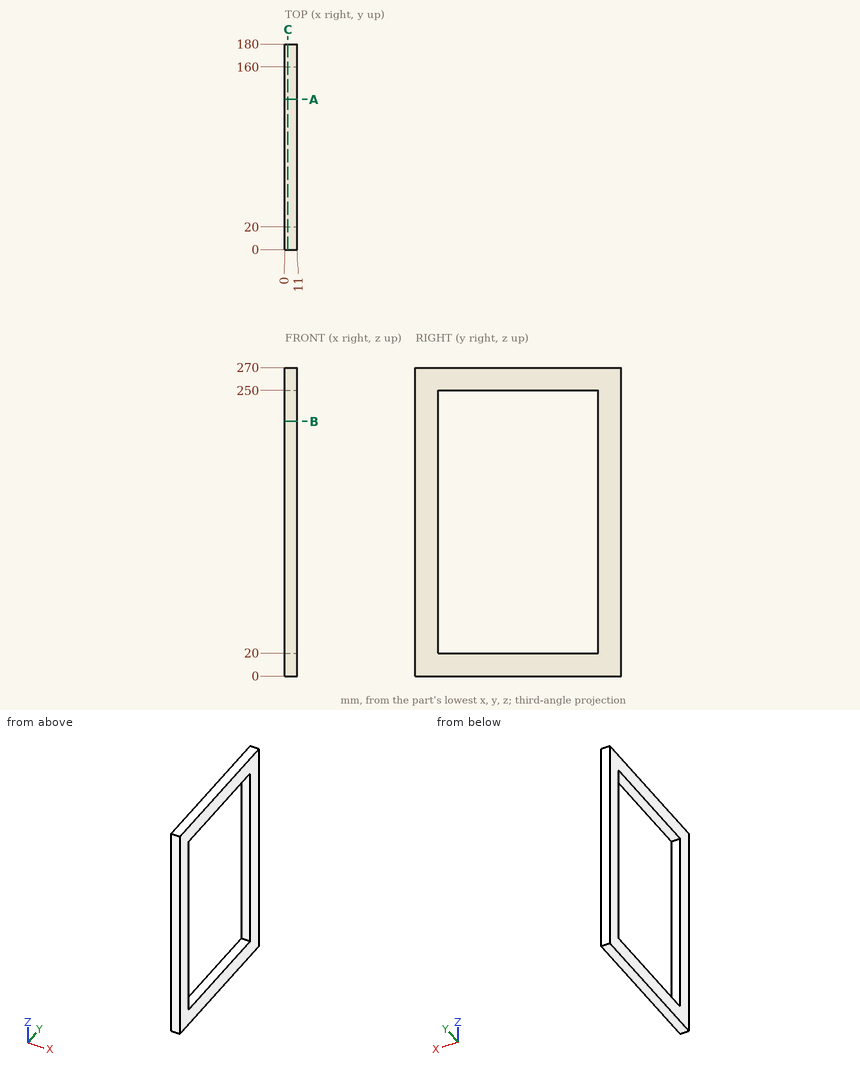
Part print with two shaded views. Sizes in mm from the minimum x, y, z corner. Round coordinates to 2 decimals unless told otherwise and drop trailing zeros. Order: outer loops, then holes, each group sorted by start corner. A loop starts at its lowest first (then second) coordinate and runs counter-clockwise, first axis right, second up. Notation, with made-up numbers: (27, 23) - (58, 23) arc R31 ccw to (58, 53) - close; hole circle Ø8 at (31.25, 62.25). An arc over 180 degrees is marked (long way). Answer in a Markdown table with one row per item. Add a question column.
(1) Probe L1, parallel to Z at x = 9.5, y = 116; L2, parallel to Y at x = 10, z = 138. List the from-to ranges inside material, lowest first. Write a range as [from, to].
(2) Band-saw the part on A-A on y = 131.5. List the corners of the cut face in (x, z), and give its area (3 significant figures).
(3) Band-saw the part on C-C on x = 2.5. List the corners of the cut face in (y, z), and give its area (3 significant figures).
(4) Band-saw the part on B-B on z = 223. List the corners of the cut face in (x, y).
Data:
| question | item | result |
|---|---|---|
| 1 | L1 | z = [0, 20], [250, 270] |
| 1 | L2 | y = [0, 20], [160, 180] |
| 2 | outline | (0, 0) - (11, 0) - (11, 20) - (0, 20) - close; (0, 250) - (11, 250) - (11, 270) - (0, 270) - close |
| 2 | area | 440 mm^2 |
| 3 | outline | (0, 0) - (180, 0) - (180, 270) - (0, 270) - close; hole (20, 20) - (160, 20) - (160, 250) - (20, 250) - close |
| 3 | area | 16,400 mm^2 |
| 4 | outline | (0, 0) - (11, 0) - (11, 20) - (0, 20) - close; (0, 160) - (11, 160) - (11, 180) - (0, 180) - close |
